Geometry check sheet. Reference: the model listing, model coordinates, mm. A direction names the side the tool comes from. Coordinates: 2 decimals unless noted, no trailing zeros. Order: outer loops, then holes, each group sorted by start corner. A loop starts at its lowest first (then second) coordinate and runs counter-clockwise, first axis right, second up. Notation, with made-up numbers: (17, 66.25) - (67, 66.25) arc R17 cw to (67, 81.25) - close; hole circle Ø1 at (78.5, -5.5). An arc over 180 degrees is marked (long way). One line per item, written item: value. Start each with the question number.
```python
from build123d import *

# Parameters (mm, degrees)
PAD_DEPTH    = 5
PAD001_DEPTH = 29
SKETCH002_W  = 52.3
SKETCH002_H  = 29.470448
POCKET_DEPTH = 24
PAD002_DEPTH = 34
SKETCH004_R  = 18.25
PAD003_DEPTH = 20
SKETCH005_R  = 16.029802
PAD004_DEPTH = 32.3
SKETCH006_R  = 5
PAD005_DEPTH = 10


with BuildPart() as part:
    # Sketch → Pad (new body)
    with BuildSketch(Plane.XZ):
        with BuildLine():
            Line((29, 0), (29, 46.4))
            ThreePointArc((29, 46.4), (27.184062, 50.784062), (22.8, 52.6))
            Line((22.8, 52.6), (-22.8, 52.6))
            ThreePointArc((-22.8, 52.6), (-27.184062, 50.784062), (-29, 46.4))
            Line((-29, 46.4), (-29, 0))
            Line((-29, 0), (29, 0))
        make_face()
        with BuildLine():
            ThreePointArc((-10.75, 39.568911), (-12.5, 46.1), (-14.25, 39.568911))
            Line((-14.25, 39.568911), (-14.25, 35.6))
            ThreePointArc((-14.25, 35.6), (-12.5, 33.85), (-10.75, 35.6))
            Line((-10.75, 35.6), (-10.75, 39.568911))
        make_face(mode=Mode.SUBTRACT)
        with BuildLine():
            ThreePointArc((14.25, 39.568911), (12.5, 46.1), (10.75, 39.568911))
            Line((10.75, 39.568911), (10.75, 35.6))
            ThreePointArc((10.75, 35.6), (12.5, 33.85), (14.25, 35.6))
            Line((14.25, 35.6), (14.25, 39.568911))
        make_face(mode=Mode.SUBTRACT)
    extrude(amount=-PAD_DEPTH)

    # Sketch001 → Pad001 (join, symmetric)
    with BuildSketch(Plane.YZ):
        Polygon((0, 0), (57.3, 0), (57.3, 2), (0, 21), align=None)
    extrude(amount=PAD001_DEPTH, both=True)

    # Sketch002 → Pocket (cut, symmetric)
    with BuildSketch(Plane.YZ):
        with Locations((31.15, 16.735224)):
            Rectangle(SKETCH002_W, SKETCH002_H)
    extrude(amount=POCKET_DEPTH, both=True, mode=Mode.SUBTRACT)

    # Sketch003 → Pad002 (join)
    with BuildSketch(Plane.XY):
        with BuildLine():
            ThreePointArc((-13.084524, 53.215476), (-21.535534, 55.835534), (-18.915476, 47.384524))
            ThreePointArc((-18.915476, 47.384524), (-23, 34.3), (-18.915476, 21.215476))
            ThreePointArc((-18.915476, 21.215476), (-21.535534, 12.764466), (-13.084524, 15.384524))
            ThreePointArc((-13.084524, 15.384524), (0, 11.3), (13.084524, 15.384524))
            ThreePointArc((13.084524, 15.384524), (21.535534, 12.764466), (18.915476, 21.215476))
            ThreePointArc((18.915476, 21.215476), (23, 34.3), (18.915476, 47.384524))
            ThreePointArc((18.915476, 47.384524), (21.535534, 55.835534), (13.084524, 53.215476))
            ThreePointArc((13.084524, 53.215476), (0, 57.3), (-13.084524, 53.215476))
        make_face()
    extrude(amount=-PAD002_DEPTH)

    # Sketch004 (on Face30 of Pad002) → Pad003 (join)
    with BuildSketch(Plane(origin=(0, 0, 2), x_dir=(-1, 0, 0), z_dir=(0, 0, 1))):
        with Locations((0, -40.224388)):
            Circle(SKETCH004_R)
    extrude(amount=PAD003_DEPTH)

    # Sketch005 (on Face44 of Pad003) → Pad004 (join)
    with BuildSketch(Plane(origin=(0, 0, 22), x_dir=(-1, 0, 0), z_dir=(0, 0, 1))):
        with Locations((0, -40.224388)):
            Circle(SKETCH005_R)
    extrude(amount=PAD004_DEPTH)

    # Sketch006 (on Face11 of Pad004) → Pad005 (join, symmetric)
    with BuildSketch(Plane(origin=(0, 57.3, 0), x_dir=(1, 0, 0), z_dir=(0, 1, 0))):
        with Locations((-7.5, 17.241444)):
            Circle(SKETCH006_R)
        with Locations((7.5, 17.241444)):
            Circle(SKETCH006_R)
    extrude(amount=PAD005_DEPTH, both=True)


solid = part.part
```
Q1. Cross-section at C-C, the plane z = -11. Enter the section's corners in (x, y), and give its area (3 significant figures).
Q2. Set-up check for faces 1 (the flat face through (0, 57.3, 1)), 2 (the flat face through (0, 2, 52.6)), 3 (the flat face through (-1.3, 56.4, 22)): record each of +Z, -Z, +X, -X, +Y, -Y from which the full face is reachable in a straight line by a thin tool's end or side.
Q3. Cross-section at D-D, the plane x = -7.5. Enter the section's corners in (y, z).
Q4. Gauge pin test, flat ends, axial feed: P1, Ø4, axis at x = 0.5, y = 1.5, coming from the +Z side; P2, Ø6.5, axis at x = 12.5, z = 42.6, coming from the +Y side; P3, Ø2, axis at y = 44, z = -12, coming from the -X side; P4, Ø1.5, axis at x = 1.5, y = 59.5, coming from the -Z side. Record the tip position at first contact, or that the pin passes through.
Q5. Material ranges on probe 1 along X at (y, z) = (49, 4); probe 2 along X at (y, z) = (1.1, 42.6); probe 3 along X at (y, z) = (9.5, 3), recorded low to high.
Q6. Release check for a two-part mould opening along Y. For faces 4 (the flat face through (24, 19, 7)), 5 (the flat face through (0, 5, 28)), 6 (the flat face through (7, 67.3, -17)), 7 (the cylindrical face through (-21.43, 55.94, -16.76)) record: released by +Y, released by -Y, zero draft, split by the parting line, or undercut.
Q7. Cross-section at A-A, the plane z = 42.6. Enter the section's corners in (x, y).
Q8. Cross-section at B-B, the plane z = 17. Enter the section's corners in (x, y), and give its area (3 significant figures).
Check result:
1. outline: (-18.92, 21.22) arc R5 ccw (long way) to (-13.08, 15.38) arc R23 ccw to (13.08, 15.38) arc R5 ccw (long way) to (18.92, 21.22) arc R23 ccw to (18.92, 47.38) arc R5 ccw (long way) to (13.08, 53.22) arc R23 ccw to (-13.08, 53.22) arc R5 ccw (long way) to (-18.92, 47.38) arc R23 ccw to start
1. area: 1,920 mm2
2. face 1: +X, -X, +Y
2. face 2: +Z, +X, -X, -Y
2. face 3: +Z
3. outline: (0, 0) - (12.56, 0) - (12.56, -34) - (56.04, -34) - (56.04, -22.24) - (67.3, -22.24) - (67.3, -12.24) - (56.04, -12.24) - (56.04, 0) - (57.3, 0) - (57.3, 2) - (56.86, 2) - (56.86, 22) - (54.39, 22) - (54.39, 54.3) - (26.06, 54.3) - (26.06, 22) - (23.59, 22) - (23.59, 2) - (5, 2) - (5, 52.6) - (0, 52.6) - close
4. P1: stops at z = 52.6
4. P2: stops at y = 53.32
4. P3: stops at x = -21.29
4. P4: passes through
5. probe 1: x = -29 to -24, -16 to 16, 24 to 29
5. probe 2: x = -29 to -16, -9 to 9, 16 to 29
5. probe 3: x = -29 to -24, 24 to 29
6. face 4: zero draft
6. face 5: undercut
6. face 6: released by +Y
6. face 7: undercut
7. outline: (-29, 0) - (-16, 0) - (-16, 5) - (-29, 5) - close; circle Ø32.06 at (0, 40.22); (-9, 0) - (9, 0) - (9, 5) - (-9, 5) - close; (16, 0) - (29, 0) - (29, 5) - (16, 5) - close
8. outline: (-29, 0) - (29, 0) - (29, 12.06) - (24, 12.06) - (24, 5) - (-24, 5) - (-24, 12.06) - (-29, 12.06) - close; circle Ø36.5 at (0, 40.22)
8. area: 1,410 mm2
